Autodesk Inventor part; units mm, degrees
ref_plane "YZ Plane" through (0, 0, 0) normal (1, 0, 0) x (0, 1, 0)
ref_plane "XZ Plane" through (0, 0, 0) normal (0, 1, 0) x (-1, 0, 0)
ref_plane "XY Plane" through (0, 0, 0) normal (0, 0, 1) x (1, 0, 0)
sketch "Boceto1" plane through (0, 0, 0) normal (0, 0, 1) x (1, 0, 0)
  circle A0 centre (0, 0) radius 3
  dimension "d0" = 6
extrude "Extrusión1" add sketch "Boceto1" along normal blind 16
sketch "Boceto2" plane through (0, 0, 16) normal (0, 0, 1) x (1, 0, 0)
  circle A0 centre (0, 0) radius 10
  dimension "d3" = 20
extrude "Extrusión2" add sketch "Boceto2" along normal blind 2
sketch "Boceto3" plane through (0, 0, 18) normal (0, 0, 1) x (1, 0, 0)
  circle A0 centre (0, 0) radius 3
  line L0 (6, 0) -> (3, -5.1962)
  line L1 (3, -5.1962) -> (-3, -5.1962)
  line L2 (-3, -5.1962) -> (-6, 0)
  line L3 (-6, 0) -> (-3, 5.1962)
  line L4 (-3, 5.1962) -> (3, 5.1962)
  line L5 (3, 5.1962) -> (6, 0)
  dimension "d6" = 6
extrude "Extrusión3" add sketch "Boceto3" along normal blind 6 contours A0 | L0 L1 L2 L3 L4 L5
sketch "Boceto4" plane through (0, 0, 24) normal (0, 0, 1) x (1, 0, 0)
  circle A0 centre (0, 0) radius 3
  dimension "d9" = 6
extrude "Extrusión4" add sketch "Boceto4" along normal blind 18
sketch "Boceto5" plane through (0, 0, 0) normal (1, 0, 0) x (0, 1, 0)
  line L0 (3, 42) -> (-3, 42)
  line L1 (-3, 24) -> (3, 24)
  arc A0 (0, 28) -> (0, 38) centre (0, 33) ccw
  line L2 (3, 24) -> (3, 42)
  line L3 (-3, 24) -> (-3, 42)
  line L4 (0, 43.0217) -> (0, 25.7964)
  point P0 (0, 0)
  point P1 (3, 33)
  point P2 (0, 24)
  dimension "d12" = 10
revolve "Revolución1" add sketch "Boceto5" angle 360 about axis through (0, 0, 43.0217) along (0, 0, -1) contours L2 A0 L4 | A0 L2
properties part number "front_plate_screw"
Work out the finished part from the listing and answer in its coordinate system (mm). A direction names the side the tool comes from. Give positions to 0.01 mm unless a question says otherwise; leave off trailing zeros. Write each loop counter-clockwise with the first axis right and the second up, starting at its lowest first coordinate (ties: lowest second). Pieces come first, ordered by that corner, then holes.
Q1. The part is cut by section A-A on y = -3.75. Give the vertices of the cut face in (x, z), and give its area (3 significant figures).
Answer:
outline: (-9.27, 16) - (9.27, 16) - (9.27, 18) - (3.83, 18) - (3.83, 24) - (-3.83, 24) - (-3.83, 18) - (-9.27, 18) - close; circle Ø6.61 at (0, 33)
area: 117 mm2
Q2. The part is cut by section D-D on z = 4. Give the vertices of the cut face in (x, y), and give its area (3 significant figures).
Answer:
outline: circle Ø6 at (0, 0)
area: 28.3 mm2
Q3. Given pin 1 (1.5 mm diameter, centred on y = 3.5, z = 22.5, fed in from -X); pin 2 (6 mm diameter, centred on x = 3, y = -5.5, fed in from -Z); pin 3 (5 mm diameter, centred on x = -7, z = 16, fed in from +Y), each flat-ended and moving along its own axis, determine where each tip first touches the part or whether it passes through.
Answer:
pin 1: stops at x = -4.41
pin 2: stops at z = 16
pin 3: stops at y = 8.93
Q4. For a pull along Z with two mould halves and no side action, classify faces 1 (the face through (0, 5.196, 21)), 2 (the face through (0, 0, 42)), 3 (the face through (3, 2, 24)), 4 (the face through (0, 0, 0)) as released by +Z, released by -Z, zero draft, split by the parting line, or undercut.
Answer:
face 1: zero draft
face 2: released by +Z
face 3: undercut
face 4: released by -Z
Q5. The part is cut by section C-C on y = 1. Give the vertices of the cut face in (x, z).
Answer:
outline: (-9.95, 16) - (-2.83, 16) - (-2.83, 0) - (2.83, 0) - (2.83, 16) - (9.95, 16) - (9.95, 18) - (5.42, 18) - (5.42, 24) - (2.83, 24) - (2.83, 29) arc R4.9 ccw to (2.83, 37) - (2.83, 42) - (-2.83, 42) - (-2.83, 37) arc R4.9 ccw to (-2.83, 29) - (-2.83, 24) - (-5.42, 24) - (-5.42, 18) - (-9.95, 18) - close
Q6. Straight lines are drawn through the part: L1, parallel to Z at x = 8, y = 5.75; L2, parallel to X at y = 0, z = 39.5; L3, parallel to Z at x = 4, y = 0. For each, find the intervals that lie inside material, in ascending order.
Answer:
L1: z = 16 to 18
L2: x = -3 to 3
L3: z = 16 to 24, 30 to 36
Q7. A tool of negligible diameter and unlimited length cuts with its end or side. For faces 5 (the face through (0, -5.196, 21)), 6 (the face through (2.1, 2.4, 16)), 7 (the face through (-4.5, -2.6, 21)), 8 (the face through (4.5, -2.6, 21)), 9 (the face through (-3, 0, 39)), from which of +Z, -Z, +X, -X, +Y, -Y can it reach the whole face along a straight path? Write none if from no direction.
Answer:
face 5: +Z, +X, -X, -Y
face 6: -Z
face 7: +Z, -X, -Y
face 8: +Z, +X, -Y
face 9: +Z
Q8. The part is cut by section B-B on x = 0. Give the vertices of the cut face in (y, z).
Answer:
outline: (-10, 16) - (-3, 16) - (-3, 0) - (3, 0) - (3, 16) - (10, 16) - (10, 18) - (5.2, 18) - (5.2, 24) - (3, 24) - (3, 29) arc R5 ccw to (3, 37) - (3, 42) - (-3, 42) - (-3, 37) arc R5 ccw to (-3, 29) - (-3, 24) - (-5.2, 24) - (-5.2, 18) - (-10, 18) - close
